Input: part model. Units: mm. Frame: model coordinates. Face numbers are marked on the shaded views. A direction names the side the tool comes from. Coordinates: 2 decimals unless noted, no trailing zeros. Loops run counter-clockwise (first coordinate to the right, second up) from the corner with the lowest first, then second, coordinate; pieces in that order, holes last. Notation, with made-up numbers: M 31,-26 L 78,-26 A24 cw 78,11 Z; hole C 10.5,30 d7. An arc over 180 degrees is marked long. Use a Markdown table: item, result. Add a question column.
1. Section B-B on y = 50.5. Output: boundary loops of the cut face in (x, z).
2. Line query: L1, parallel to X at y = 20, z = 0; L2, parallel to Z at x = 53, y = 13; L3, parallel to Z at x = 0, y = 35. Output: solid intervals per line, ascending. Write a range as [from, to].
3. Pin query (flat end, axial travel): pin 1 (5 mm diameter, centred on x = -19, z = -14, fed in from -Y); pin 2 (10 mm diameter, centred on x = 56.5, y = 35, fed in from +Z); pin 3 (2 mm diameter, centred on y = 21, z = 25, fed in from -X). Return the tip coordinate at first contact, or that it passes through.
4. Set-up query: the marked faces 4, 5 and 6. Return all of +Z, -Z, +X, -X, +Y, -Y with unobstructed straight access to the full face (end or side cutting, diameter ignored); none if empty.
5. Draft query along X for the marked faces 1, 2 and 3. Return one class per face: +X half, -X half, draft (parallel to the pull), parting line (faces both ways), or undercut.
6. Section A-A on x = 129. Output: boundary loops of the cut face in (y, z).
7. Section C-C on z = 0. Output: boundary loops of the cut face in (x, y).
```python
from build123d import *
from build123d.topology import SkipClean

# Parameters (mm, degrees)
SALIENTE_EXTRUIR1_DEPTH = 65
SALIENTE_EXTRUIR2_DEPTH = 2.5
CROQUIS4_W              = 101
CROQUIS4_H              = 10
CORTAR_EXTRUIR1_DEPTH   = 250
SALIENTE_EXTRUIR3_DEPTH = 3


with BuildPart() as part:
    # Croquis2 → Saliente-Extruir1 (new body)
    with BuildSketch(Plane(origin=(0, 0, 0), x_dir=(1, 0, 0), z_dir=(0, 1, 0))):
        with BuildLine():
            Line((151, 39.865398531), (31, 39.865398531))
            ThreePointArc((31, 39.865398531), (-50.499518563, 0.220510468), (30.650673156, -40.134601469))
            Line((30.650673156, -40.134601469), (151, -40.134601469))
            Line((151, -40.134601469), (151, 39.865398531))
        make_face()
        with BuildLine():
            Line((30.655028903, 38.865398531), (150, 38.865398531))
            Line((150, 38.865398531), (150, -39.134601469))
            Line((150, -39.134601469), (30.310608173, -39.134601469))
            ThreePointArc((30.310608173, -39.134601469), (-49.499517432, 0.218572563), (30.655028903, 38.865398531))
        make_face(mode=Mode.SUBTRACT)
    extrude(amount=SALIENTE_EXTRUIR1_DEPTH)

    # Croquis3 → Saliente-Extruir2 (add)
    with SkipClean():  # the faces are left unmerged after this step: merging them gives an invalid solid
        with BuildSketch(Plane(origin=(0, 65, 0), x_dir=(1, 0, 0), z_dir=(0, 1, 0))):
            with BuildLine():
                Line((151, 39.865398531), (151, -40.134601469))
                Line((151, -40.134601469), (30.650673156, -40.134601469))
                ThreePointArc((30.650673156, -40.134601469), (-50.499518563, 0.220510468), (31, 39.865398531))
                Line((31, 39.865398531), (151, 39.865398531))
            make_face()
        extrude(amount=SALIENTE_EXTRUIR2_DEPTH)

    # Croquis4 → Cortar-Extruir1 (cut)
    with BuildSketch(Plane(origin=(151, 0, 0), x_dir=(0, 0, -1), z_dir=(1, 0, 0))):
        with Locations((0, 62.5)):
            Rectangle(CROQUIS4_W, CROQUIS4_H)
    extrude(amount=-CORTAR_EXTRUIR1_DEPTH, mode=Mode.SUBTRACT)

    # Croquis5 → Saliente-Extruir3 (add)
    with BuildSketch(Plane(origin=(0, 57.5, 0), x_dir=(1, 0, 0), z_dir=(0, 1, 0))):
        with BuildLine():
            Line((151, 39.865398531), (31, 39.865398531))
            ThreePointArc((31, 39.865398531), (-50.499518563, 0.220510468), (30.650673156, -40.134601469))
            Line((30.650673156, -40.134601469), (151, -40.134601469))
            Line((151, -40.134601469), (151, 39.865398531))
        make_face()
    extrude(amount=SALIENTE_EXTRUIR3_DEPTH)


solid = part.part
```
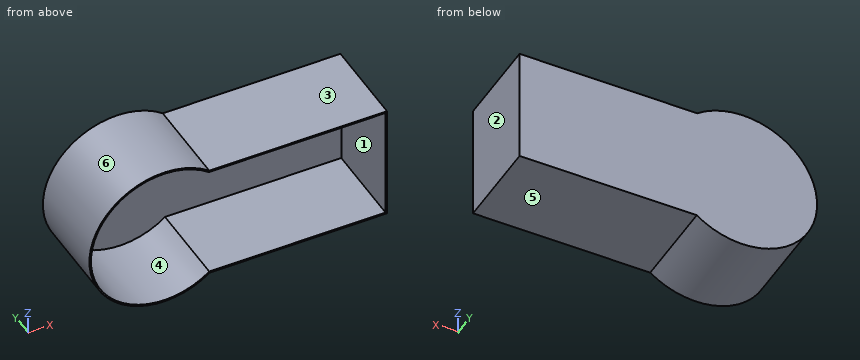
Answers below:
| question | item | result |
|---|---|---|
| 1 | outline | M 30.65,40.13 A50.5 ccw long 31,-39.87 L 151,-39.87 L 151,40.13 Z; hole M 30.31,39.13 A49.5 ccw long 30.66,-38.87 L 150,-38.87 L 150,39.13 Z |
| 2 | L1 | x = [-50.5, -49.5], [150, 151] |
| 2 | L2 | z = [-39.87, -38.87], [39.13, 40.13] |
| 2 | L3 | z = [-50.5, -49.5], [49.5, 50.5] |
| 3 | pin 1 | stops at y = 57.5 |
| 3 | pin 2 | stops at z = 40.13 |
| 3 | pin 3 | stops at x = -44.43 |
| 4 | face 4 | -Y |
| 4 | face 5 | -Z, +X, +Y, -Y |
| 4 | face 6 | +Y, -Y |
| 5 | face 1 | undercut |
| 5 | face 2 | +X half |
| 5 | face 3 | draft |
| 6 | outline | M 0,-39.87 L 60.5,-39.87 L 60.5,40.13 L 0,40.13 L 0,39.13 L 57.5,39.13 L 57.5,-38.87 L 0,-38.87 Z |
| 7 | outline | M -50.5,0 L -49.5,0 L -49.5,57.5 L 150,57.5 L 150,0 L 151,0 L 151,60.5 L -50.5,60.5 Z |
